```python
from build123d import *

# Parameters (mm, degrees)
SKETCH7_W            = 100
SKETCH7_H            = 100
BOSS_EXTRUDE2_DEPTH  = 10
SKETCH8_W            = 100
SKETCH8_H            = 100
SKETCH8_W_2          = 90
SKETCH8_H_2          = 90
BOSS_EXTRUDE3_DEPTH  = 50
CHAMFER1_SIZE        = 10
CUT_EXTRUDE5_DEPTH   = 15
FILLET3_R            = 1
SKETCH16_W           = 30
SKETCH16_H           = 30
CUT_EXTRUDE6_DEPTH   = 10
SKETCH17_W           = 6
SKETCH17_H           = 6
SKETCH17_R           = 1.7
BOSS_EXTRUDE4_DEPTH  = 5
LPATTERN2_COUNT      = 2
LPATTERN2_PITCH      = 24
LPATTERN2_COUNT_DIR2 = 2
LPATTERN2_PITCH_DIR2 = 24
SKETCH18_R           = 2.5
CUT_EXTRUDE7_DEPTH   = 10
LPATTERN3_COUNT      = 2
LPATTERN3_PITCH      = 30
LPATTERN3_COUNT_DIR2 = 2
LPATTERN3_PITCH_DIR2 = 50
SKETCH19_W           = 20
SKETCH19_H           = 60
CUT_EXTRUDE8_DEPTH   = 10
SKETCH20_R           = 1.5
CUT_EXTRUDE9_DEPTH   = 5
LPATTERN4_COUNT      = 2
LPATTERN4_PITCH      = 95
LPATTERN4_COUNT_DIR2 = 2
LPATTERN4_PITCH_DIR2 = 95


with BuildPart() as part:
    # Sketch7 → Boss-Extrude2 (new body)
    with BuildSketch(Plane(origin=(0, 0, 0), x_dir=(0, 0, -1), z_dir=(1, 0, 0))):
        Rectangle(SKETCH7_W, SKETCH7_H)
    extrude(amount=BOSS_EXTRUDE2_DEPTH)

    # Sketch8 → Boss-Extrude3 (add)
    with BuildSketch(Plane(origin=(10, 0, 0), x_dir=(0, 0, -1), z_dir=(1, 0, 0))):
        Rectangle(SKETCH8_W, SKETCH8_H)
        Rectangle(SKETCH8_W_2, SKETCH8_H_2, mode=Mode.SUBTRACT)
    extrude(amount=BOSS_EXTRUDE3_DEPTH)

    # Chamfer1
    chamfer1_edges = [part.edges().sort_by_distance(p)[0] for p in [
        (0, 50, 0),
        (0, 0, -50),
        (0, -50, 0),
        (0, 0, 50),
    ]]
    chamfer(chamfer1_edges, length=CHAMFER1_SIZE)

    # Sketch14 → Cut-Extrude5 (cut)
    with BuildSketch(Plane.ZY):
        with BuildLine():
            Line((-25, 37.5), (25, 37.5))
            ThreePointArc((25, 37.5), (30, 32.5), (25, 27.5))
            Line((25, 27.5), (-25, 27.5))
            ThreePointArc((-25, 27.5), (-30, 32.5), (-25, 37.5))
        make_face()
    extrude(amount=-CUT_EXTRUDE5_DEPTH, mode=Mode.SUBTRACT)

    # Fillet3
    fillet3_edges = [part.edges().sort_by_distance(p)[0] for p in [
        (10, 27.5, 0),
        (10, 32.5, 30),
        (10, 37.5, 0),
        (10, 32.5, -30),
        (0, 32.5, -30),
        (0, 27.5, 0),
        (0, 32.5, 30),
        (0, 37.5, 0),
    ]]
    fillet(fillet3_edges, radius=FILLET3_R)

    # Sketch16 → Cut-Extrude6 (cut)
    with BuildSketch(Plane.XZ.offset(50)):
        with Locations((30, 0)):
            Rectangle(SKETCH16_W, SKETCH16_H)
    extrude(amount=-CUT_EXTRUDE6_DEPTH, mode=Mode.SUBTRACT)

    # Sketch17 → Boss-Extrude4 (add)
    with BuildSketch(Plane.XZ.offset(50)):
        with Locations((18, 12)):
            Rectangle(SKETCH17_W, SKETCH17_H)
        with Locations((18, 12)):
            Circle(SKETCH17_R, mode=Mode.SUBTRACT)
    boss_extrude4 = extrude(amount=-BOSS_EXTRUDE4_DEPTH)

    # LPattern2: Boss-Extrude4 2 × 2
    with Locations(*[(i * LPATTERN2_PITCH, 0, -j * LPATTERN2_PITCH_DIR2) for i in range(LPATTERN2_COUNT) for j in range(LPATTERN2_COUNT_DIR2) if (i, j) != (0, 0)]):
        add(boss_extrude4)

    # Sketch18 → Cut-Extrude7 (cut)
    with BuildSketch(Plane.ZY):
        with Locations((-15, 20)):
            Circle(SKETCH18_R)
    cut_extrude7 = extrude(amount=-CUT_EXTRUDE7_DEPTH, mode=Mode.SUBTRACT)

    # LPattern3: Cut-Extrude7 2 × 2
    with Locations(*[(0, -j * LPATTERN3_PITCH_DIR2, i * LPATTERN3_PITCH) for i in range(LPATTERN3_COUNT) for j in range(LPATTERN3_COUNT_DIR2) if (i, j) != (0, 0)]):
        add(cut_extrude7, mode=Mode.SUBTRACT)

    # Sketch19 → Cut-Extrude8 (cut)
    with BuildSketch(Plane.XY.offset(50)):
        with Locations((50, 5)):
            Rectangle(SKETCH19_W, SKETCH19_H)
    extrude(amount=-CUT_EXTRUDE8_DEPTH, mode=Mode.SUBTRACT)

    # Sketch20 → Cut-Extrude9 (cut)
    with BuildSketch(Plane(origin=(60, 0, 0), x_dir=(0, 0, -1), z_dir=(1, 0, 0))):
        with Locations((-47.5, 47.5)):
            Circle(SKETCH20_R)
    cut_extrude9 = extrude(amount=-CUT_EXTRUDE9_DEPTH, mode=Mode.SUBTRACT)

    # LPattern4: Cut-Extrude9 2 × 2
    with Locations(*[(0, -j * LPATTERN4_PITCH_DIR2, -i * LPATTERN4_PITCH) for i in range(LPATTERN4_COUNT) for j in range(LPATTERN4_COUNT_DIR2) if (i, j) != (0, 0)]):
        add(cut_extrude9, mode=Mode.SUBTRACT)


solid = part.part
```
Source: CAD feature listing. Evaluate the final solid. Frame: model axes, mm. A direction names the side the tool comes from. Give positions to 0.01 mm unless a question says otherwise; leave off trailing zeros. Order: outer loops, then holes, each group sorted by start corner. A loop starts at its lowest first (then second) coordinate and runs counter-clockwise, first axis right, second up.
(1) Access query for faces 4 (the face through (4.9, 32.6, 30)), 5 (the face through (19.57, -47.54, 11.35)), 6 (the face through (35, 45, 1)). Directions: +Z, -Z, +X, -X, +Y, -Y. A direction counts if a zero-diameter tool reaches every point of the face in a straight line with its end or side. Return the directions, or none.
(2) Section query C-C (y = -47.5). State how many separate pieces and enclosed holes the cut face has, plus the area to 3 significant figures.
(3) Material intervals for line 1 along Y through (x, z) = (56.25, 47.5); line 2 along Z through (x, y) = (18, -46.3); line 3 along Z through (x, y) = (37, -18.5), sorted ascending.
(4) Contact query for flat-ended pins moving along their axis: P1, Ø2.5, axis at x = 6.5, z = 4, coming from the -Y side; P2, Ø10, axis at y = 3, z = 19, coming from the +X side; P3, Ø2.5, axis at x = 42, z = -12, coming from the -Y side. Output: stop coordinate, or through.
(5) Pull-direction query (Y, two-part tool) for faces 1 (the face through (21, -48, 12)), 2 (the face through (5, 45, 1)), 3 (the face through (5, 27.5, 0)); classes: +Y half, -Y half, draft (parallel to the pull), parting line (faces both ways), or undercut.
(6) Section query B-B (z = -6). Return the cut outline in (x, y).
(7) Section query A-A (x = 18). Return the cut outline in (y, z), plus the area to 3 significant figures.
(8) Section query D-D (z = -47.5). Return the cut outline in (x, y), plus the area to 3 significant figures.
Outcome:
1. face 4: +X, -X
1. face 5: -Y
1. face 6: +X
2. separate pieces: 1
2. enclosed holes: 5
2. area: 4,420 mm2
3. line 1: y = -50 to -49, -46 to -25, 35 to 46, 49 to 50
3. line 2: z = -50 to -13.7, -10.3 to -9, 9 to 10.3, 13.7 to 50
3. line 3: z = -50 to -45, 45 to 50
4. P1: stops at y = -47.75
4. P2: stops at x = 10
4. P3: stops at y = 45
5. face 1: draft
5. face 2: +Y half
5. face 3: undercut
6. outline: (0, -40) - (10, -50) - (15, -50) - (15, -45) - (10, -45) - (10, 26.5) arc R1 ccw to (9, 27.5) - (1, 27.5) arc R1 ccw to (0, 26.5) - close; (0, 38.5) arc R1 ccw to (1, 37.5) - (9, 37.5) arc R1 ccw to (10, 38.5) - (10, 45) - (60, 45) - (60, 50) - (10, 50) - (0, 40) - close; (45, -50) - (60, -50) - (60, -45) - (45, -45) - close
7. outline: (-50, -50) - (50, -50) - (50, 50) - (-50, 50) - (-50, 13.7) - (-45, 13.7) - (-45, 45) - (45, 45) - (45, -45) - (-45, -45) - (-45, -13.7) - (-50, -13.7) - close; (-50, -10.3) - (-45, -10.3) - (-45, -9) - (-50, -9) - close; (-50, 9) - (-45, 9) - (-45, 10.3) - (-50, 10.3) - close
7. area: 1,780 mm2
8. outline: (7.5, -47.5) - (10, -50) - (60, -50) - (60, -49) - (55, -49) - (55, -46) - (60, -46) - (60, 46) - (55, 46) - (55, 49) - (60, 49) - (60, 50) - (10, 50) - (7.5, 47.5) - close
8. area: 5,210 mm2
